```python
from build123d import *

# Parameters (mm, degrees)
CYLINDER003_R     = 2
CYLINDER003_DEPTH = 10
CYLINDER002_R     = 2
CYLINDER002_DEPTH = 10
CYLINDER001_R     = 2
CYLINDER001_DEPTH = 10
CYLINDER_R        = 62
CYLINDER_DEPTH    = 3
CHAMFER_SIZE      = 2
CHAMFER001_SIZE   = 1
CHAMFER002_SIZE   = 1
CHAMFER003_SIZE   = 1


with BuildPart() as cylinder003:
    # Cylinder003 → Cylinder003 (new body)
    with BuildSketch(Plane(origin=(-46, 27, 0), x_dir=(1, 0, 0), z_dir=(0, 0, 1))):
        Circle(CYLINDER003_R)
    extrude(amount=CYLINDER003_DEPTH)


with BuildPart() as cylinder002:
    # Cylinder002 → Cylinder002 (new body)
    with BuildSketch(Plane(origin=(46, 27, 0), x_dir=(1, 0, 0), z_dir=(0, 0, 1))):
        Circle(CYLINDER002_R)
    extrude(amount=CYLINDER002_DEPTH)


with BuildPart() as cylinder001:
    # Cylinder001 → Cylinder001 (new body)
    with BuildSketch(Plane(origin=(0, -55, 0), x_dir=(1, 0, 0), z_dir=(0, 0, 1))):
        Circle(CYLINDER001_R)
    extrude(amount=CYLINDER001_DEPTH)


with BuildPart() as cover_plate:
    # Cylinder → Cylinder (new body)
    with BuildSketch(Plane.XY):
        Circle(CYLINDER_R)
    extrude(amount=CYLINDER_DEPTH)

    # Cut: cut Cylinder001
    add(cylinder001.part, mode=Mode.SUBTRACT)

    # Cut001: cut Cylinder002
    add(cylinder002.part, mode=Mode.SUBTRACT)

    # Cut002: cut Cylinder003
    add(cylinder003.part, mode=Mode.SUBTRACT)

    # Chamfer
    chamfer_edges = [cover_plate.edges().sort_by_distance(p)[0] for p in [
        (-62, 0, 3),
    ]]
    chamfer(chamfer_edges, length=CHAMFER_SIZE)

    # Chamfer001
    chamfer001_edges = [cover_plate.edges().sort_by_distance(p)[0] for p in [
        (-48, 27, 3),
    ]]
    chamfer(chamfer001_edges, length=CHAMFER001_SIZE)

    # Chamfer002
    chamfer002_edges = [cover_plate.edges().sort_by_distance(p)[0] for p in [
        (44, 27, 3),
    ]]
    chamfer(chamfer002_edges, length=CHAMFER002_SIZE)

    # Chamfer003
    chamfer003_edges = [cover_plate.edges().sort_by_distance(p)[0] for p in [
        (-2, -55, 3),
    ]]
    chamfer(chamfer003_edges, length=CHAMFER003_SIZE)


solid = cover_plate.part
```
Work out the finished part from the listing and answer in its coordinate system (mm). Give positions to 0.01 mm unless a question says otherwise; leave off trailing zeros. Loops run counter-clockwise (first coordinate to the right, second up) from the corner with the lowest first, then second, coordinate; pieces in that order, holes last. Notation, with made-up numbers: (28.25, 27.5) -> (55.25, 27.5) arc R7 cw to (55.25, 33.5) -> close; hole circle Ø4 at (-8, 36.25). An arc over 180 degrees is marked (long way). One line per question, with ' | ' between items. Start each with the question number.
1) Section A-A, the plane x = 0 is taken. Determine the outline of the cut face in (y, z).
2) Determine the mould class of faces 1 (the face through (-1, 1, 3)), 2 (the face through (0, -53, 1)), 3 (the face through (-8.071, 61.472, 0.493)) for opening direction Y: +Y half, -Y half, draft (parallel to the pull), parting line (faces both ways), or undercut.
3) Section C-C, the plane y = 27 is taken. State how many separate pieces and enclosed holes the cut face has, then the cut area to 3 significant figures.
4) Straight lines are drawn through the part: L1, parallel to X at y = 27, z = 0.85; L2, parallel to Y at x = -46, z = 1.45; L3, parallel to Y at x = 46, z = 1.35. For each, find the intervals that lie inside material, in ascending order.
5) Section B-B, the plane z = 0.5 is taken. Determine the outline of the cut face in (x, y), then the cut area to 3 significant figures.
6) Each of these flat-tipped pins is pushed along its axis until it touches: pin 1 (1 mm diameter, centred on y = 45.5, z = 1, fed in from -X); pin 2 (10 mm diameter, centred on x = 44, y = -13.5, fed in from -Z); pin 3 (1 mm diameter, centred on y = 23, z = 1, fed in from +X); pin 4 (4 mm diameter, centred on x = 38.5, y = 49.5, fed in from +Z). Where does it stop, or does it pass through?
Resolved:
1) outline: (-62, 0) -> (-57, 0) -> (-57, 2) -> (-58, 3) -> (-60, 3) -> (-62, 1) -> close; (-53, 0) -> (62, 0) -> (62, 1) -> (60, 3) -> (-52, 3) -> (-53, 2) -> close
2) face 1: draft | face 2: undercut | face 3: parting line
3) separate pieces: 3 | enclosed holes: 0 | area: 304 mm2
4) L1: -55.81 to -48, -44 to 44, 48 to 55.81 | L2: -40.9 to 25, 29 to 40.9 | L3: -41.05 to 25, 29 to 41.05
5) outline: circle Ø124 at (0, 0); hole circle Ø4 at (-46, 27); hole circle Ø4 at (0, -55); hole circle Ø4 at (46, 27) | area: 12,000 mm2
6) pin 1: x = -42.65 | pin 2: z = 0 | pin 3: x = 57.77 | pin 4: z = 2.29
